```python
from build123d import *

# Parameters (mm, degrees)
ESQUISSE1_R             = 11
ESQUISSE1_R_2           = 4
BASE_EXTRUSION_DEPTH    = 7
ESQUISSE2_R             = 9.5
ESQUISSE2_R_2           = 6
ENL_V_MAT_EXTRU_1_DEPTH = 0.5
ENL_V_START             = -0.5
ESQUISSE3_R             = 9.5
ESQUISSE3_R_2           = 6
ENL_V_MAT_EXTRU_2_DEPTH = 0.5
CHANFREIN1_SIZE         = 0.5


with BuildPart() as part:
    # Esquisse1 → Base-Extrusion (new body)
    with BuildSketch(Plane.XY):
        Circle(ESQUISSE1_R)
        Circle(ESQUISSE1_R_2, mode=Mode.SUBTRACT)
    extrude(amount=BASE_EXTRUSION_DEPTH)

    # Esquisse2 → Enlèv. mat.-Extru.1 (cut)
    with BuildSketch(Plane.XY.offset(7)):
        Circle(ESQUISSE2_R)
        Circle(ESQUISSE2_R_2, mode=Mode.SUBTRACT)
    extrude(amount=-ENL_V_MAT_EXTRU_1_DEPTH, mode=Mode.SUBTRACT)

    # Esquisse3 → Enlèv. mat.-Extru.2 (cut)
    with BuildSketch(Plane(origin=(0, 0, 0), x_dir=(-1, 0, 0), z_dir=(0, 0, -1)).offset(ENL_V_START)):
        with Locations(Location((0, 0, 0), (0, 0, 180))):
            Circle(ESQUISSE3_R)
        with Locations(Location((0, 0, 0), (0, 0, 180))):
            Circle(ESQUISSE3_R_2, mode=Mode.SUBTRACT)
    extrude(amount=ENL_V_MAT_EXTRU_2_DEPTH, mode=Mode.SUBTRACT)

    # Chanfrein1
    chanfrein1_edges = [part.edges().sort_by_distance(p)[0] for p in [
        (-9.5, 0, 7),
        (-6, 0, 7),
        (-9.5, 0, 0),
        (-6, 0, 0),
        (-11, 0, 0),
        (-11, 0, 7),
        (-4, 0, 0),
        (-4, 0, 7),
    ]]
    chamfer(chanfrein1_edges, length=CHANFREIN1_SIZE - 0.0001)  # a hair under: the kernel refuses the full size


solid = part.part
```
Model file for the job. Use its own axes, mm. A direction names the side the tool comes from. Give positions to 0.01 mm unless a question says otherwise; leave off trailing zeros. Write each loop counter-clockwise with the first axis right and the second up, starting at its lowest first coordinate (ties: lowest second). Pieces come first, ordered by that corner, then holes. Notation, with made-up numbers: (32.25, -22) -> (57.25, -22) arc R17 cw to (57.25, -3) -> close; hole circle Ø8 at (-32.5, 9). An arc over 180 degrees is marked (long way). Use CSV: the item, a comma, the result in double quotes. Start each with the question number.
1) Tool access for faces 4 (the cylindrical face through (-0.867, -3.905, 3.458)), 5 (the flat face through (-0.1, 6.2, 0.5)): list every direction of +Z, -Z, +X, -X, +Y, -Y with a clear straight run to the whole face (end or side of a thin tool).
2) Cut at A-A on z = 4.75. List the corners of the cut face in (x, y), plus the area to 3 significant figures.
3) Two-plate mould, pull along X, no slides. Class faces 1 (the cylindrical face through (-2.38, -10.74, 3.46)), 2 (the flat face through (5, -9, 7)), 3 (the flat face through (-0.1, -6.2, 6.5)): released by +X, released by -X, zero draft, split by the parting line, or undercut.
4) Drill centre lines: L1, parallel to Z at x = -5, y = -4.75; L2, parallel to Y at x = -0.75, z = 2.75; L3, parallel to X at y = -9, z = 6. Where is each one in solid material? Low to high.
5) Pin check, flat tips, straight feed: P1, Ø4, axis at y = -8, z = 3.5, coming from the +X side; P2, Ø1.5, axis at y = 5.5, z = 4, coming from the +X side; P3, Ø1.5, axis at y = -4.5, z = 2, coming from the +X side. Stop position of each tip, or through.
Final values:
1,face 4,"+Z, -Z"
1,face 5,"-Z"
2,outline,"circle Ø22 at (0, 0); hole circle Ø8 at (0, 0)"
2,area,"330 mm2"
3,face 1,"split by the parting line"
3,face 2,"zero draft"
3,face 3,"undercut"
4,L1,"z = 0.5 to 6.5"
4,L2,"y = -10.97 to -3.93, 3.93 to 10.97"
4,L3,"x = -6.32 to 6.32"
5,P1,"stops at x = 9.22"
5,P2,"stops at x = 9.92"
5,P3,"stops at x = 10.34"
